```python
from build123d import *

# Parameters (mm, degrees)
SKETCH_W              = 40.5
SKETCH_H              = 40.5
PAD_DEPTH             = 25.5
SKETCH001_R           = 9
PAD001_DEPTH          = 1.8
POLARPATTERN_COUNT    = 2
POLARPATTERN_ANGLE    = 90
SKETCH002_R           = 2.5
POCKET_DEPTH          = 5
POLARPATTERN001_COUNT = 2
POLARPATTERN001_ANGLE = 90
SKETCH003_R           = 2.5
SKETCH003_R_2         = 1.19
POCKET001_DEPTH       = 5
POCKET002_DEPTH       = 5
FILLET_R              = 4
FILLET001_R           = 2


with BuildPart() as part:
    # Sketch → Pad (new body)
    with BuildSketch(Plane.XY):
        Rectangle(SKETCH_W, SKETCH_H)
    extrude(amount=PAD_DEPTH)

    # Sketch001 (on Face3 of Pad) → Pad001 (join)
    with BuildSketch(Plane.XZ.offset(20.25)):
        with Locations((0, 16.5)):
            Circle(SKETCH001_R)
    pad001 = extrude(amount=PAD001_DEPTH)

    # PolarPattern: Pad001 ×2 about axis
    polarpattern_axis = Axis((0, 0, 0), (0, 0, 1))
    for i in range(1, POLARPATTERN_COUNT):
        add(pad001.rotate(polarpattern_axis, i * POLARPATTERN_ANGLE / (POLARPATTERN_COUNT - 1)))

    # Sketch002 (on Face10 of PolarPattern) → Pocket (cut)
    with BuildSketch(Plane.XZ.offset(22.05)):
        with Locations((0, 16.5)):
            Circle(SKETCH002_R)
    pocket = extrude(amount=-POCKET_DEPTH, mode=Mode.SUBTRACT)

    # PolarPattern001: Pocket ×2 about axis
    polarpattern001_axis = Axis((0, 0, 0), (0, 0, 1))
    for i in range(1, POLARPATTERN001_COUNT):
        add(pocket.rotate(polarpattern001_axis, i * POLARPATTERN001_ANGLE / (POLARPATTERN001_COUNT - 1)), mode=Mode.SUBTRACT)

    # Sketch003 (on Face5 of PolarPattern001) → Pocket001 (cut)
    with BuildSketch(Plane.XY.offset(25.5)):
        Circle(SKETCH003_R)
        with Locations((-16.015969, 16.015969)):
            Circle(SKETCH003_R_2)
        with Locations((16.015969, 16.015969)):
            Circle(SKETCH003_R_2)
        with Locations((-16.015969, -16.015969)):
            Circle(SKETCH003_R_2)
        with Locations((16.015969, -16.015969)):
            Circle(SKETCH003_R_2)
    extrude(amount=-POCKET001_DEPTH, mode=Mode.SUBTRACT)

    # Sketch003 (on Face5 of PolarPattern001) → Pocket002 (cut)
    with BuildSketch(Plane.XY.offset(25.5)):
        Circle(SKETCH003_R)
        with Locations((-16.015969, 16.015969)):
            Circle(SKETCH003_R_2)
        with Locations((16.015969, 16.015969)):
            Circle(SKETCH003_R_2)
        with Locations((-16.015969, -16.015969)):
            Circle(SKETCH003_R_2)
        with Locations((16.015969, -16.015969)):
            Circle(SKETCH003_R_2)
    extrude(amount=-POCKET002_DEPTH, mode=Mode.SUBTRACT)

    # Fillet
    fillet_edges = [part.edges().sort_by_distance(p)[0] for p in [
        (20.25, 20.25, 12.75),
        (20.25, -20.25, 12.75),
        (-20.25, -20.25, 12.75),
        (-20.25, 20.25, 12.75),
    ]]
    fillet(fillet_edges, radius=FILLET_R)

    # Fillet001
    fillet001_edges = [part.edges().sort_by_distance(p)[0] for p in [
        (0, 20.25, 0),
        (-19.078427, 19.078427, 0),
        (19.078427, 19.078427, 0),
        (-20.25, 0, 0),
        (20.25, 0, 0),
        (-19.078427, -19.078427, 0),
        (19.078427, -19.078427, 0),
        (0, -20.25, 0),
    ]]
    fillet(fillet001_edges, radius=FILLET001_R)


solid = part.part
```
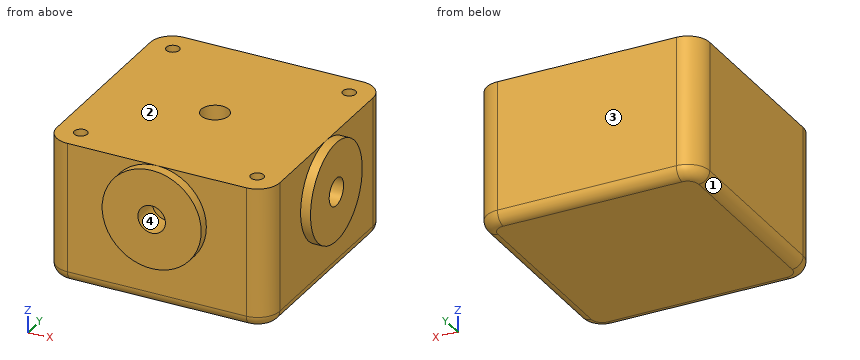
Input: part model. Units: mm. Frame: model coordinates. Face numbers are marked on the shaded views. Give positions to 0.01 mm unless a question says otherwise; leave off trailing zeros. Write each loop counter-clockwise with the first axis right and the second up, starting at its lowest first coordinate (ties: lowest second). Pieces come first, ordered by that corner, then holes. Notation, with made-up numbers: (20.5, 74.5) - (51.5, 74.5) arc R30 cw to (51.5, 99.5) - close; hole circle Ø8 at (85.25, 89.25). An arc over 180 degrees is marked (long way). Write item = value, one per line. Start each with the question number.
1) Cut plane C-C (y = 5). Return loops of the section in (x, z).
2) Cut plane A-A (z = 5.25). Return loops of the section in (x, y).
3) Pin query (flat end, axial travel): pin 1 (1.9 mm diameter, centred on x = 15.5, y = 15.5, fed in from +Z); pin 2 (0.7 mm diameter, centred on x = -16.5, y = 16, fed in from +Z); pin 3 (1.5 mm diameter, centred on y = 1, z = 17.5, fed in from +X). Return the tip coordinate at first contact, or that it passes through.
4) Material intervals for L1, parallel to Z at x = 20.3, y = 0; L2, parallel to Y at x = 1, z = 5.5, sorted ascending. Write a range as [from, to].
5) Draft query along Z for the marked faces 1, 2, 3 and 4. Return one class per face: pulls with the +Z half, pulls with the -Z half, needs draft (parallel to the pull), parting line crosses it, or undercut.
6) Cut plane D-D (z = 16.5). Return loops of the section in (x, y), and give its area (3 significant figures).
7) Cut plane B-B (x = 13). Return loops of the section in (y, z), and give its area (3 significant figures).
Answers follow:
q1.outline = (-20.25, 2) arc R2 ccw to (-18.25, 0) - (18.25, 0) arc R2 ccw to (20.25, 2) - (20.25, 9.02) - (22.05, 9.02) - (22.05, 23.98) - (20.25, 23.98) - (20.25, 25.5) - (-20.25, 25.5) - close
q2.outline = (-20.25, -16.25) arc R4 ccw to (-16.25, -20.25) - (16.25, -20.25) arc R4 ccw to (20.25, -16.25) - (20.25, 16.25) arc R4 ccw to (16.25, 20.25) - (-16.25, 20.25) arc R4 ccw to (-20.25, 16.25) - close
q3.pin_1 = 25.5
q3.pin_2 = 20.5
q3.pin_3 = 17.05
q4.L1 = [7.5, 14], [19, 25.5]
q4.L2 = [-20.25, 20.25]
q5.face_1 = pulls with the -Z half
q5.face_2 = pulls with the +Z half
q5.face_3 = needs draft
q5.face_4 = undercut
q6.outline = (-20.25, -16.25) arc R4 ccw to (-16.25, -20.25) - (-9, -20.25) - (-9, -22.05) - (-2.5, -22.05) - (-2.5, -17.05) - (2.5, -17.05) - (2.5, -22.05) - (9, -22.05) - (9, -20.25) - (16.25, -20.25) arc R4 ccw to (20.25, -16.25) - (20.25, -9) - (22.05, -9) - (22.05, -2.5) - (17.05, -2.5) - (17.05, 2.5) - (22.05, 2.5) - (22.05, 9) - (20.25, 9) - (20.25, 16.25) arc R4 ccw to (16.25, 20.25) - (-16.25, 20.25) arc R4 ccw to (-20.25, 16.25) - close
q6.area = 1,640 mm^2
q7.outline = (-20.25, 2) arc R2 ccw to (-18.25, 0) - (18.25, 0) arc R2 ccw to (20.25, 2) - (20.25, 25.5) - (-20.25, 25.5) - close
q7.area = 1,030 mm^2
